Input: part model. Units: mm. Frame: model coordinates. Coordinates: 2 decimals unless noted, no trailing zeros. Order: outer loops, then holes, each group sorted by start corner. A loop starts at its lowest first (then second) coordinate and runs counter-clockwise, first axis right, second up. Notation, with made-up numbers: (-38.75, 31) - (13.25, 31) arc R11 cw to (13.25, 50) - close; hole circle Ø10 at (70.5, -3.5). An arc over 180 degrees is marked (long way). Answer as CSV lines item,"result". Start each with the question number.
Item 1: Section B-B (y = -8.5). Output: boundary loops of the cut face in (x, z).
Item 2: Section A-A (x = 25). Output: boundary loops of the cut face in (y, z), and give its area (3 significant figures).
Item 3: First-contact query: pin 1 (14 mm diameter, centred on x = 20.92, z = 231.41, fed in from -Y); pin 2 (20 mm diameter, centred on x = 229.08, z = 231.41, fed in from +Y). Flat tips, straight axial feed; report the tip coordinate or a pass-through.
Item 4: Material intervals for line 1 along X through (y, z) = (-12, 14.5); line 2 along X through (y, z) = (-9.75, 21.5); line 3 along Z through (x, y) = (22.5, -0.75), sorted ascending.
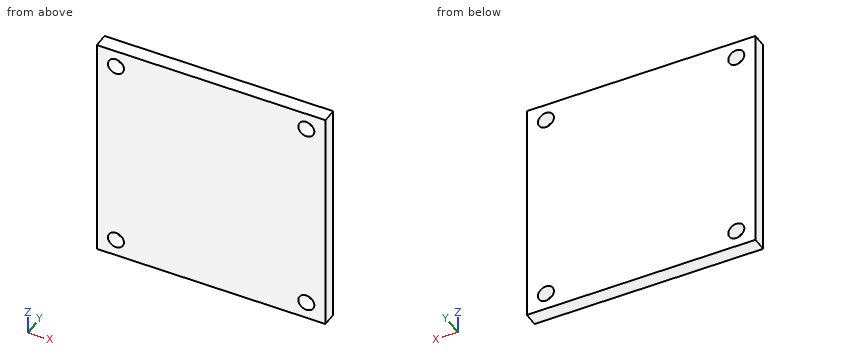
from build123d import *

# Parameters (mm, degrees)
F0_W     = 250
F0_H     = 250
F1_DEPTH = 16
F3_D     = 17.5


with BuildPart() as f1:
    # F0 (on Front) → F1 (new body)
    with BuildSketch(Plane.XZ):
        with Locations((125, 125)):
            Rectangle(F0_W, F0_H)
    extrude(amount=F1_DEPTH)

    # F3 (through all)
    with Locations(Plane.XZ.offset(16)):
        with Locations((20.9212601185, 231.4076423645), (20.9212601185, 18.5923576355), (229.0787398815, 18.5923576355), (229.0787398815, 231.4076423645)):
            Hole(F3_D / 2)


solid = f1.part
Determined:
1,outline,"(0, 0) - (250, 0) - (250, 250) - (0, 250) - close; hole circle Ø17.5 at (20.92, 18.59); hole circle Ø17.5 at (20.92, 231.41); hole circle Ø17.5 at (229.08, 18.59); hole circle Ø17.5 at (229.08, 231.41)"
2,outline,"(-16, 0) - (0, 0) - (0, 10.85) - (-16, 10.85) - close; (-16, 26.33) - (0, 26.33) - (0, 223.67) - (-16, 223.67) - close; (-16, 239.15) - (0, 239.15) - (0, 250) - (-16, 250) - close"
2,area,"3,500 mm^2"
3,pin 1,"passes through"
3,pin 2,"stops at y = 0"
4,line 1,"x = 0 to 13.19, 28.66 to 221.34, 236.81 to 250"
4,line 2,"x = 0 to 12.67, 29.17 to 220.83, 237.33 to 250"
4,line 3,"z = 0 to 9.99, 27.2 to 222.8, 240.01 to 250"
